from build123d import *

# Parameters (mm, degrees)
SKETCH1_W            = 76.2
SKETCH1_H            = 38.1
BOSS_EXTRUDE1_DEPTH  = 6.35
M6_CLEARANCE_HOLE1_D = 7
CHAMFER1_SIZE        = 2.54


with BuildPart() as part:
    # Sketch1 → Boss-Extrude1 (new body)
    with BuildSketch(Plane(origin=(0, 0, 0), x_dir=(1, 0, 0), z_dir=(0, 1, 0))):
        Rectangle(SKETCH1_W, SKETCH1_H)
    extrude(amount=BOSS_EXTRUDE1_DEPTH)

    # M6 Clearance Hole1 (through all)
    with Locations(Plane(origin=(0, 6.35, 0), x_dir=(1, 0, 0), z_dir=(0, 1, 0))):
        with Locations((-22.999999974, 0), (22.999999974, 0)):
            Hole(M6_CLEARANCE_HOLE1_D / 2)

    # Chamfer1
    chamfer1_edges = [part.edges().sort_by_distance(p)[0] for p in [
        (38.1, 3.175, 19.05),
        (-38.1, 3.175, 19.05),
        (-38.1, 3.175, -19.05),
        (38.1, 3.175, -19.05),
    ]]
    chamfer(chamfer1_edges, length=CHAMFER1_SIZE)


solid = part.part
The listing builds one solid part. Answer for the finished solid, in the listing's coordinates (mm). Give positions to 0.01 mm unless a question says otherwise; leave off trailing zeros. Loops run counter-clockwise (first coordinate to the right, second up) from the corner with the lowest first, then second, coordinate; pieces in that order, holes last. Notation, with made-up numbers: (-33.75, 3.5) - (-12.75, 3.5) arc R9 cw to (-12.75, 16.5) - close; hole circle Ø11 at (17, 14.25). An arc over 180 degrees is marked (long way). Answer as a JSON object with one key per item and string values.
1. A cutting plane is placed at B-B (z = 0). Write down the section's boundary in (x, y), then the cut area to 3 significant figures.
Determined:
{"outline": "(-38.1, 0) - (-26.5, 0) - (-26.5, 6.35) - (-38.1, 6.35) - close; (-19.5, 0) - (19.5, 0) - (19.5, 6.35) - (-19.5, 6.35) - close; (26.5, 0) - (38.1, 0) - (38.1, 6.35) - (26.5, 6.35) - close", "area": "395 mm²"}
2. For a pull along Z with two mould halves and no side action, classify faces 1 (the flat face through (-38.1, 3, 0)), 2 (the flat face through (-36.81, 3.13, -17.8)), 3 (the cylindrical face through (19.66, 3.13, -1.05)), 4 (the flat face through (36.85, 3.13, 17.76)) as pulls with the +Z half, pulls with the -Z half, needs draft (parallel to the pull), parting line crosses it, or undercut.
Determined:
{"face 1": "needs draft", "face 2": "pulls with the -Z half", "face 3": "undercut", "face 4": "pulls with the +Z half"}
3. Flat-ended cylindrical pins translate along their axes: pin 1 Ø10 at (x, z) = (-20, 6) entering from -Y; pin 2 Ø4 at (x, z) = (23, 0) entering from +Y. Find the tip coordinate at first contact, or state that the pin passes through.
Determined:
{"pin 1": "y = 0", "pin 2": "through"}
4. A cutting plane is placed at C-C (x = -23). Write down the section's boundary in (y, z).
Determined:
{"outline": "(0, -19.05) - (6.35, -19.05) - (6.35, -3.5) - (0, -3.5) - close; (0, 3.5) - (6.35, 3.5) - (6.35, 19.05) - (0, 19.05) - close"}
5. Find the intervals of material crossed by L1, parallel to Z at x = -23, y = 4; L2, parallel to Z at x = -20, y = 5; L3, parallel to X at y = 0.5, z = 17, in increasing order. Write a range as [from, to].
Determined:
{"L1": "[-19.05, -3.5], [3.5, 19.05]", "L2": "[-19.05, -1.8], [1.8, 19.05]", "L3": "[-37.61, 37.61]"}
6. A cutting plane is placed at A-A (y = 2.75). Write down the section's boundary in (x, z).
Determined:
{"outline": "(-38.1, -16.51) - (-35.56, -19.05) - (35.56, -19.05) - (38.1, -16.51) - (38.1, 16.51) - (35.56, 19.05) - (-35.56, 19.05) - (-38.1, 16.51) - close; hole circle Ø7 at (-23, 0); hole circle Ø7 at (23, 0)"}
